Verification items for the finished model (mm, model axes). A direction names the side the tool comes from. Coordinates: 2 decimals unless noted, no trailing zeros. Order: outer loops, then holes, each group sorted by start corner. A loop starts at its lowest first (then second) coordinate and runs counter-clockwise, first axis right, second up. Notation, with made-up numbers: M 3.25,-32 L 18.25,-32 A26 ccw 18.25,-17 Z; hole C 52,50 d7. An arc over 180 degrees is marked long. Answer as a JSON object with one key per item and string values. Group by question number.
(1) Material ranges on line 1 (Y direction, x = 0, z = 30); line 2 (X direction, y = -0.5, z = 58); line 3 (X direction, y = 21, z = 13), recorded low to high.
(2) Gauge pin test, flat ends, axial feed: pin 1 Ø3.5 at (x, y) = (0.5, 0.5) entering from -Z; pin 2 Ø4 at (x, z) = (-2, 47.5) entering from -Y; pin 3 Ø4 at (x, z) = (0, 18) entering from +Y; pin 4 Ø4 at (y, z) = (6.5, 19.5) entering from +X. Record the tip position at first contact, or that the pin passes through.
(3) Cross-section at C-C (z = 43). Enter the section's corners in (x, y).
(4) Cross-section at D-D (z = 5). Enter the section's corners in (x, y) (1 decimal).
(5) Cross-section at A-A (x = 0). Enter the section's corners in (y, z).
(6) Access from +Z, -Z, +X, -X, +Y, -Y to the whole of each face (thin tool, end or side, straight path). Record for faces 4 (the face through (0, 5, 62.274)), 5 (the face through (-3.78, -2.9, 57.58)), 6 (the face through (0, 0, 21.844)).
(7) Mould release check, pull along Y, two halves, no side actions. Record for faces 1 (the face through (-1.582, 7.126, 46.464)), 2 (the face through (6, 6, 30.207)), 3 (the face through (-0.34, -1.55, 10.79)): released by +Y, released by -Y, zero draft, split by the parting line, or undercut.
from build123d import *

# Parameters (mm, degrees)
F2_R     = 4.7625
F3_DEPTH = 9.525
F4_R     = 1.5875
F5_DEPTH = 21.844


with BuildPart() as f1:
    # F0 (on Front) → F1 (revolve)
    with BuildSketch(Plane.XZ):
        with BuildLine():
            Line((0, 62.27351), (0, 0))
            ThreePointArc((0, 0), (21.359254, 8.847293), (30.206546, 30.206546))
            Line((30.206546, 30.206546), (7.299625, 30.206546))
            Line((7.299625, 30.206546), (7.299625, 62.27351))
            Line((7.299625, 62.27351), (0, 62.27351))
        make_face()
    revolve(axis=Axis((0, 0, 31.136755), (0, 0, -1)))

    # F2 (on face) → F3 (cut)
    with BuildSketch(Plane.XY.offset(62.27351)):
        Circle(F2_R)
    extrude(amount=-F3_DEPTH, mode=Mode.SUBTRACT)

    # F4 (on Top) → F5 (cut)
    with BuildSketch(Plane.XY):
        Circle(F4_R)
    extrude(amount=F5_DEPTH, mode=Mode.SUBTRACT)


solid = f1.part
Taken from the geometry:
{
 "1": {"line 1": "y = -30.21 to 30.21", "line 2": "x = -7.28 to -4.74, 4.74 to 7.28", "line 3": "x = -13.24 to 13.24"},
 "2": {"pin 1": "stops at z = 0.04", "pin 2": "stops at y = -7.3", "pin 3": "stops at y = 28.43", "pin 4": "stops at x = 28.31"},
 "3": {"outline": "C 0,0 d14.6"},
 "4": {"outline": "C 0,0 d33.3; hole C 0,0 d3.2"},
 "5": {"outline": "M -30.21,30.21 A30.21 ccw -1.59,0.04 L -1.59,21.84 L 1.59,21.84 L 1.59,0.04 A30.21 ccw 30.21,30.21 L 7.3,30.21 L 7.3,62.27 L 4.76,62.27 L 4.76,52.75 L -4.76,52.75 L -4.76,62.27 L -7.3,62.27 L -7.3,30.21 Z"},
 "6": {"face 4": "+Z, +X, -X, +Y, -Y", "face 5": "+Z", "face 6": "-Z"},
 "7": {"face 1": "split by the parting line", "face 2": "zero draft", "face 3": "undercut"}
}
